Work out the finished part from the listing and answer in its coordinate system (mm). Round coordinates to 2 decimals unless told otherwise and drop trailing zeros. Order: outer loops, then holes, each group sorted by start corner. A loop starts at its lowest first (then second) coordinate and runs counter-clockwise, first axis right, second up. Notation, with made-up numbers: (-17.75, -36.5) - (33.25, -36.5) arc R21 cw to (33.25, -27.5) - close; hole circle Ø4 at (51, 64). An arc over 180 degrees is marked (long way). Put each result on its own line as item: value.
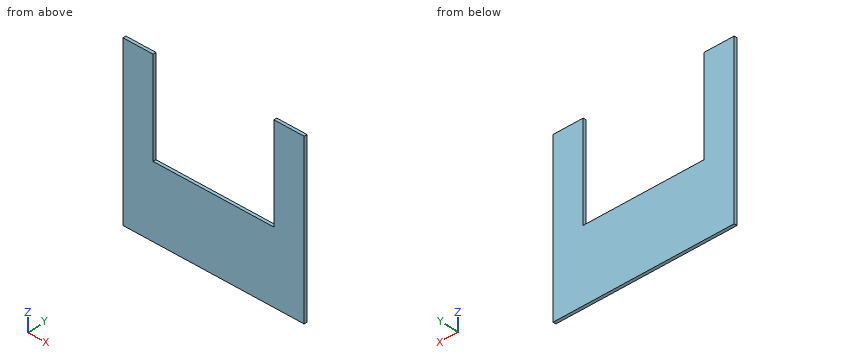
```python
from build123d import *

# Parameters (mm, degrees)
SKETCH1_W           = 381
SKETCH1_H           = 429.26
BOSS_EXTRUDE1_DEPTH = 6.35
SKETCH2_W           = 254
SKETCH2_H           = 203.2
CUT_EXTRUDE1_DEPTH  = 6.35
SKETCH3_W           = 381
SKETCH3_H           = 73.66
CUT_EXTRUDE2_DEPTH  = 6.35
SKETCH4_W           = 254
SKETCH4_H           = 6.35
CUT_EXTRUDE3_DEPTH  = 73.66


with BuildPart() as part:
    # Sketch1 → Boss-Extrude1 (new body)
    with BuildSketch(Plane(origin=(0, 0, 0), x_dir=(1, 0, 0), z_dir=(0, 1, 0))):
        with Locations((190.5, 214.63)):
            Rectangle(SKETCH1_W, SKETCH1_H)
    extrude(amount=BOSS_EXTRUDE1_DEPTH)

    # Sketch2 → Cut-Extrude1 (cut)
    with BuildSketch(Plane(origin=(0, 6.35, 0), x_dir=(1, 0, 0), z_dir=(0, 1, 0))):
        with Locations((190.5, 101.6)):
            Rectangle(SKETCH2_W, SKETCH2_H)
    extrude(amount=-CUT_EXTRUDE1_DEPTH, mode=Mode.SUBTRACT)

    # Sketch3 → Cut-Extrude2 (cut)
    with BuildSketch(Plane(origin=(0, 6.35, 0), x_dir=(1, 0, 0), z_dir=(0, 1, 0))):
        with Locations((190.5, 36.83)):
            Rectangle(SKETCH3_W, SKETCH3_H)
    extrude(amount=-CUT_EXTRUDE2_DEPTH, mode=Mode.SUBTRACT)

    # Sketch4 → Cut-Extrude3 (cut)
    with BuildSketch(Plane.XY.offset(-203.2)):
        with Locations((190.5, 3.175)):
            Rectangle(SKETCH4_W, SKETCH4_H)
    extrude(amount=-CUT_EXTRUDE3_DEPTH, mode=Mode.SUBTRACT)


solid = part.part
```
1) Given pin 1 Ø1.9 at (y, z) = (2.5, -163.5) entering from -X; pin 2 Ø3 at (x, y) = (175, 4) entering from +Z, each flat-ended and moving along its own axis, determine where each tip first touches the part or whether it passes through.
Findings below:
pin 1: stops at x = 0
pin 2: stops at z = -276.86
2) A cutting plane is placed at C-C on x = 193. Write down the section's boundary in (y, z), then the cut area to 3 significant figures.
Findings below:
outline: (0, -429.26) - (6.35, -429.26) - (6.35, -276.86) - (0, -276.86) - close
area: 968 mm2
3) A cutting plane is placed at A-A on z = -107. Write down the section's boundary in (x, y), then the cut area to 3 significant figures.
Findings below:
outline: (0, 0) - (63.5, 0) - (63.5, 6.35) - (0, 6.35) - close; (317.5, 0) - (381, 0) - (381, 6.35) - (317.5, 6.35) - close
area: 806 mm2
4) A cutting plane is placed at B-B on y = 3.75. Write down the section's boundary in (x, z).
Findings below:
outline: (0, -429.26) - (381, -429.26) - (381, -73.66) - (317.5, -73.66) - (317.5, -276.86) - (63.5, -276.86) - (63.5, -73.66) - (0, -73.66) - close
5) Straight lines are drawn through the part: L1, parallel to X at y = 1.5, z = -214; L2, parallel to Z at x = 167, y = 2.25. For each, find the intervals that lie inside material, in ascending order. Write a range as from..to.
Findings below:
L1: x = 0..63.5, 317.5..381
L2: z = -429.26..-276.86
